Design review of the part built by this model. Coordinates are the model's own, in mm. A direction names the side the tool comes from. Coordinates: 2 decimals unless noted, no trailing zeros. Write each loop counter-clockwise with the first axis right and the second up, starting at its lowest first coordinate (ties: lowest second). Pieces come first, ordered by that corner, then holes. Notation, with made-up numbers: M 87.25,-5 L 92.25,-5 A15 ccw 92.25,8 Z; hole C 71.25,70 d1. An arc over 180 degrees is marked long. Write each question's results on one line, items separated by ' | '. Start each with the question number.
```python
from build123d import *

# Parameters (mm, degrees)
SKETCH1_R           = 12.7
SKETCH1_R_2         = 5.588
BOSS_EXTRUDE1_DEPTH = 2.54


with BuildPart() as part:
    # Sketch1 → Boss-Extrude1 (new body)
    with BuildSketch(Plane(origin=(0, 0, 0), x_dir=(1, 0, 0), z_dir=(0, 1, 0))):
        with Locations(Location((0, 0, 0), (0, 0, 270))):
            Circle(SKETCH1_R)
        with Locations(Location((0, 0, 0), (0, 0, 270))):
            Circle(SKETCH1_R_2, mode=Mode.SUBTRACT)
        with BuildLine():
            Line((-9.68793232, 5.043218354), (-6.759022549, 3.518524433))
            ThreePointArc((-6.759022549, 3.518524433), (-6.974673471, 3.068929777), (-7.16045777, 2.606193492))
            Line((-7.16045777, 2.606193492), (-10.263322804, 3.735544005))
            ThreePointArc((-10.263322804, 3.735544005), (-9.997031975, 4.398799347), (-9.68793232, 5.043218354))
        make_face(mode=Mode.SUBTRACT)
        with BuildLine():
            Line((-8.606653451, 6.724254634), (-6.004641942, 4.691340442))
            ThreePointArc((-6.004641942, 4.691340442), (-5.684957198, 5.074018295), (-5.340928594, 5.434968423))
            Line((-5.340928594, 5.434968423), (-7.655330985, 7.790121406))
            ThreePointArc((-7.655330985, 7.790121406), (-8.14843865, 7.272759556), (-8.606653451, 6.724254634))
        make_face(mode=Mode.SUBTRACT)
        with BuildLine():
            Line((-6.107504892, 9.054748367), (-4.261049924, 6.317266303))
            ThreePointArc((-4.261049924, 6.317266303), (-3.838757705, 6.58242655), (-3.400027336, 6.819399835))
            Line((-3.400027336, 6.819399835), (-4.873372515, 9.774473097))
            ThreePointArc((-4.873372515, 9.774473097), (-5.502219377, 9.434811388), (-6.107504892, 9.054748367))
        make_face(mode=Mode.SUBTRACT)
        with BuildLine():
            Line((-3.0105112, 10.498900243), (-2.100356651, 7.324814123))
            ThreePointArc((-2.100356651, 7.324814123), (-1.616793862, 7.446501031), (-1.126307713, 7.536300879))
            Line((-1.126307713, 7.536300879), (-1.614374388, 10.80203126))
            ThreePointArc((-1.614374388, 10.80203126), (-2.317404535, 10.673318145), (-3.0105112, 10.498900243))
        make_face(mode=Mode.SUBTRACT)
        with BuildLine():
            Line((0.381172303, 10.915346613), (0.265934165, 7.615358102))
            ThreePointArc((0.265934165, 7.615358102), (0.763433029, 7.581660109), (1.257662757, 7.515496284))
            Line((1.257662757, 7.515496284), (1.802649951, 10.77221134))
            ThreePointArc((1.802649951, 10.77221134), (1.094254009, 10.867046156), (0.381172303, 10.915346613))
        make_face(mode=Mode.SUBTRACT)
        with BuildLine():
            Line((3.735544005, 10.263322804), (2.606193492, 7.16045777))
            ThreePointArc((2.606193492, 7.16045777), (3.068929777, 6.974673471), (3.518524433, 6.759022549))
            Line((3.518524433, 6.759022549), (5.043218354, 9.68793232))
            ThreePointArc((5.043218354, 9.68793232), (4.398799347, 9.997031975), (3.735544005, 10.263322804))
        make_face(mode=Mode.SUBTRACT)
        with BuildLine():
            Line((6.724254634, 8.606653451), (4.691340442, 6.004641942))
            ThreePointArc((4.691340442, 6.004641942), (5.074018295, 5.684957198), (5.434968423, 5.340928594))
            Line((5.434968423, 5.340928594), (7.790121406, 7.655330985))
            ThreePointArc((7.790121406, 7.655330985), (7.272759556, 8.14843865), (6.724254634, 8.606653451))
        make_face(mode=Mode.SUBTRACT)
        with BuildLine():
            Line((9.054748367, 6.107504892), (6.317266303, 4.261049924))
            ThreePointArc((6.317266303, 4.261049924), (6.58242655, 3.838757705), (6.819399835, 3.400027336))
            Line((6.819399835, 3.400027336), (9.774473097, 4.873372515))
            ThreePointArc((9.774473097, 4.873372515), (9.434811388, 5.502219377), (9.054748367, 6.107504892))
        make_face(mode=Mode.SUBTRACT)
        with BuildLine():
            Line((10.498900243, 3.0105112), (7.324814123, 2.100356651))
            ThreePointArc((7.324814123, 2.100356651), (7.446501031, 1.616793862), (7.536300879, 1.126307713))
            Line((7.536300879, 1.126307713), (10.80203126, 1.614374388))
            ThreePointArc((10.80203126, 1.614374388), (10.673318145, 2.317404535), (10.498900243, 3.0105112))
        make_face(mode=Mode.SUBTRACT)
        with BuildLine():
            Line((10.915346613, -0.381172303), (7.615358102, -0.265934165))
            ThreePointArc((7.615358102, -0.265934165), (7.581660109, -0.763433029), (7.515496284, -1.257662757))
            Line((7.515496284, -1.257662757), (10.77221134, -1.802649951))
            ThreePointArc((10.77221134, -1.802649951), (10.867046156, -1.094254009), (10.915346613, -0.381172303))
        make_face(mode=Mode.SUBTRACT)
        with BuildLine():
            Line((10.263322804, -3.735544005), (7.16045777, -2.606193492))
            ThreePointArc((7.16045777, -2.606193492), (6.974673471, -3.068929777), (6.759022549, -3.518524433))
            Line((6.759022549, -3.518524433), (9.68793232, -5.043218354))
            ThreePointArc((9.68793232, -5.043218354), (9.997031975, -4.398799347), (10.263322804, -3.735544005))
        make_face(mode=Mode.SUBTRACT)
        with BuildLine():
            Line((8.606653451, -6.724254634), (6.004641942, -4.691340442))
            ThreePointArc((6.004641942, -4.691340442), (5.684957198, -5.074018295), (5.340928594, -5.434968423))
            Line((5.340928594, -5.434968423), (7.655330985, -7.790121406))
            ThreePointArc((7.655330985, -7.790121406), (8.14843865, -7.272759556), (8.606653451, -6.724254634))
        make_face(mode=Mode.SUBTRACT)
        with BuildLine():
            Line((6.107504892, -9.054748367), (4.261049924, -6.317266303))
            ThreePointArc((4.261049924, -6.317266303), (3.838757705, -6.58242655), (3.400027336, -6.819399835))
            Line((3.400027336, -6.819399835), (4.873372515, -9.774473097))
            ThreePointArc((4.873372515, -9.774473097), (5.502219377, -9.434811388), (6.107504892, -9.054748367))
        make_face(mode=Mode.SUBTRACT)
        with BuildLine():
            Line((3.0105112, -10.498900243), (2.100356651, -7.324814123))
            ThreePointArc((2.100356651, -7.324814123), (1.616793862, -7.446501031), (1.126307713, -7.536300879))
            Line((1.126307713, -7.536300879), (1.614374388, -10.80203126))
            ThreePointArc((1.614374388, -10.80203126), (2.317404535, -10.673318145), (3.0105112, -10.498900243))
        make_face(mode=Mode.SUBTRACT)
        with BuildLine():
            Line((-0.381172303, -10.915346613), (-0.265934165, -7.615358102))
            ThreePointArc((-0.265934165, -7.615358102), (-0.763433029, -7.581660109), (-1.257662757, -7.515496284))
            Line((-1.257662757, -7.515496284), (-1.802649951, -10.77221134))
            ThreePointArc((-1.802649951, -10.77221134), (-1.094254009, -10.867046156), (-0.381172303, -10.915346613))
        make_face(mode=Mode.SUBTRACT)
        with BuildLine():
            Line((-3.735544005, -10.263322804), (-2.606193492, -7.16045777))
            ThreePointArc((-2.606193492, -7.16045777), (-3.068929777, -6.974673471), (-3.518524433, -6.759022549))
            Line((-3.518524433, -6.759022549), (-5.043218354, -9.68793232))
            ThreePointArc((-5.043218354, -9.68793232), (-4.398799347, -9.997031975), (-3.735544005, -10.263322804))
        make_face(mode=Mode.SUBTRACT)
        with BuildLine():
            Line((-6.724254634, -8.606653451), (-4.691340442, -6.004641942))
            ThreePointArc((-4.691340442, -6.004641942), (-5.074018295, -5.684957198), (-5.434968423, -5.340928594))
            Line((-5.434968423, -5.340928594), (-7.790121406, -7.655330985))
            ThreePointArc((-7.790121406, -7.655330985), (-7.272759556, -8.14843865), (-6.724254634, -8.606653451))
        make_face(mode=Mode.SUBTRACT)
        with BuildLine():
            Line((-9.054748367, -6.107504892), (-6.317266303, -4.261049924))
            ThreePointArc((-6.317266303, -4.261049924), (-6.58242655, -3.838757705), (-6.819399835, -3.400027336))
            Line((-6.819399835, -3.400027336), (-9.774473097, -4.873372515))
            ThreePointArc((-9.774473097, -4.873372515), (-9.434811388, -5.502219377), (-9.054748367, -6.107504892))
        make_face(mode=Mode.SUBTRACT)
        with BuildLine():
            Line((-10.498900243, -3.0105112), (-7.324814123, -2.100356651))
            ThreePointArc((-7.324814123, -2.100356651), (-7.446501031, -1.616793862), (-7.536300879, -1.126307713))
            Line((-7.536300879, -1.126307713), (-10.80203126, -1.614374388))
            ThreePointArc((-10.80203126, -1.614374388), (-10.673318145, -2.317404535), (-10.498900243, -3.0105112))
        make_face(mode=Mode.SUBTRACT)
        with BuildLine():
            Line((-10.915346613, 0.381172303), (-7.615358102, 0.265934165))
            ThreePointArc((-7.615358102, 0.265934165), (-7.581660109, 0.763433029), (-7.515496284, 1.257662757))
            Line((-7.515496284, 1.257662757), (-10.77221134, 1.802649951))
            ThreePointArc((-10.77221134, 1.802649951), (-10.867046156, 1.094254009), (-10.915346613, 0.381172303))
        make_face(mode=Mode.SUBTRACT)
    extrude(amount=BOSS_EXTRUDE1_DEPTH)


solid = part.part
```
Item 1: We need section B-B on y = 1.95. Count the separate pieces of the cut face and the enclosed holes in it, then the cut area to 3 significant figures.
Item 2: For faces 1 (the flat face through (-3, 2.54, 5)), 2 (the flat face through (-9.146, 1.252, 1.367)), list the 3-axis set-ups (+Z, -Z, +X, -X, +Y, -Y) from which the entire face can be reached by the end or side of a thin tool; tool diameter is ignored.
Item 3: Insertion check: pin 1 Ø10 at (x, z) = (0, 0) entering from +Y. The pin has a flat end and moves straight along its axis. Give the tip position at first contact, or say it passes through.
Item 4: We need section A-A on x = -0.75. State the section outline as (y, z) points, then the cut area to 3 significant figures.
Item 5: Wall thickness on L1, parallel to X at y = 2.1, z = 8; L2, parallel to Z at x = 9.5, y = 1.6; L3, parallel to X at y = 0.85, z = 4.5: over which ranges is each line inside the solid? List them lowest first.
Answer:
1) separate pieces: 1 | enclosed holes: 21 | area: 328 mm^2
2) face 1: +Z, -Z, +X, -X, +Y | face 2: +Y, -Y
3) pin 1: passes through
4) outline: M 0,-12.68 L 2.54,-12.68 L 2.54,-5.54 L 0,-5.54 Z; M 0,5.54 L 2.54,5.54 L 2.54,7.58 L 0,7.58 Z; M 0,10.9 L 2.54,10.9 L 2.54,12.68 L 0,12.68 Z | area: 27.9 mm^2
5) L1: x = -9.86 to -7.44, -6.25 to -4.16, -2.91 to -1.34, -0.28 to 1.2, 2.29 to 3.99, 5.4 to 9.86 | L2: z = -8.43 to -5.39, -4.74 to -2.72, -1.42 to 0.33, 1.59 to 3.46, 4.95 to 8.43 | L3: x = -11.88 to -9.03, -6.67 to -3.31, 3.31 to 8.64, 9.95 to 11.88
